```python
from build123d import *

# Parameters (mm, degrees)
BOSS_EXTRUDE1_DEPTH = 6
CUT_EXTRUDE1_DEPTH  = 3.2
SKETCH4_R           = 3
SKETCH4_R_2         = 2
CUT_EXTRUDE2_DEPTH  = 2
SKETCH2_W           = 92.1
SKETCH2_H           = 8
BOSS_EXTRUDE2_DEPTH = 6
FILLET1_R           = 1


with BuildPart() as part:
    # Sketch1 → Boss-Extrude1 (new body)
    with BuildSketch(Plane(origin=(0, 0, 0), x_dir=(1, 0, 0), z_dir=(0, 1, 0))):
        with BuildLine():
            Line((-53.95, 0), (-53.95, 106.281608618))
            ThreePointArc((-53.95, 106.281608618), (-50, 118.95), (-46.05, 106.281608618))
            Line((-46.05, 106.281608618), (-46.05, 0))
            Line((-46.05, 0), (-53.95, 0))
        make_face()
    extrude(amount=BOSS_EXTRUDE1_DEPTH)

    # Sketch3 → Cut-Extrude1 (cut)
    with BuildSketch(Plane.XZ):
        with BuildLine():
            Line((-53.95, -106.281608618), (-53.95, -96.9))
            Line((-53.95, -96.9), (-46.05, -96.9))
            Line((-46.05, -96.9), (-46.05, -106.281608618))
            ThreePointArc((-46.05, -106.281608618), (-50, -118.95), (-53.95, -106.281608618))
        make_face()
    extrude(amount=-CUT_EXTRUDE1_DEPTH, mode=Mode.SUBTRACT)

    # Sketch4 → Cut-Extrude2 (cut)
    with BuildSketch(Plane.XZ.offset(-3.2)):
        with Locations(Location((-50, -112, 0), (0, 0, 270))):
            Circle(SKETCH4_R)
        with Locations(Location((-50, -102, 0), (0, 0, 270))):
            Circle(SKETCH4_R_2)
    extrude(amount=-CUT_EXTRUDE2_DEPTH, mode=Mode.SUBTRACT)


with BuildPart() as body_2:
    # Mirror3: mirrored copy
    add(part.part.mirror(Plane(origin=(0, 0, 0), x_dir=(0, 0, 1), z_dir=(1, 0, 0))))

    # Mirror4 2: body 2 across plane


with BuildPart() as part_1:
    add(part.part)

    # Mirror4: part across plane
    add(part.part.mirror(Plane.XY))



with BuildPart() as body_2_1:
    add(body_2.part)
    add(body_2.part.mirror(Plane.XY))


with BuildPart() as part_2:
    add(part_1.part)

    add(body_2_1.part)  # Boss-Extrude2 merges body 2
    # Sketch2 → Boss-Extrude2 (add)
    with BuildSketch(Plane(origin=(0, 6, 0), x_dir=(1, 0, 0), z_dir=(0, 1, 0))):
        with Locations((0, 54)):
            Rectangle(SKETCH2_W, SKETCH2_H)
        with Locations((0, -54)):
            Rectangle(SKETCH2_W, SKETCH2_H)
    extrude(amount=-BOSS_EXTRUDE2_DEPTH)

    # Fillet1
    fillet1_edges = [part_2.edges().sort_by_distance(p)[0] for p in [
        (-46.05, 0, 0),
        (-46.05, 6, 0),
        (46.05, 3, 50),
        (46.05, 3, 58),
        (-46.05, 3, 58),
        (-46.05, 3, 50),
        (0, 6, 50),
        (0, 6, 58),
        (0, 0, 58),
        (0, 0, 50),
        (-53.95, 0, 0),
        (-53.95, 6, 0),
        (-46.05, 0, 77.45),
        (-46.05, 0, -77.45),
        (-46.05, 6, -82.140804309),
        (-46.05, 3, -50),
        (-46.05, 3, -58),
        (46.05, 3, -58),
        (46.05, 3, -50),
        (0, 6, -50),
        (0, 6, -58),
        (0, 0, -58),
        (0, 0, -50),
        (46.05, 6, -82.140804309),
        (46.05, 6, 82.140804309),
        (53.95, 6, 0),
        (53.95, 0, 0),
        (46.05, 0, 77.45),
        (46.05, 0, -77.45),
        (-46.05, 6, 82.140804309),
        (46.05, 0, 0),
        (46.05, 6, 0),
    ]]
    fillet(fillet1_edges, radius=FILLET1_R)


solid = part_2.part
```
The model under review builds one solid part; all positions refer to its coordinate system, in mm. A direction names the side the tool comes from. Round coordinates to 2 decimals unless told otherwise and drop trailing zeros. Order: outer loops, then holes, each group sorted by start corner. A loop starts at its lowest first (then second) coordinate and runs counter-clockwise, first axis right, second up.
(1) For P1, Ø1, axis at y = 5, z = 6.5, coming from the +X side; P2, Ø2, axis at y = 1, z = 69, coming from the -X side; P3, Ø3, axis at x = 49.5, z = -111.5, coming from the -Y side; P4, Ø8, axis at x = 40.5, z = -85.5, coming from the +Y side, all flat-tipped, find the tip position at first contact; note any pin that passes through.
Working result:
P1: stops at x = 53.95
P2: stops at x = -53.95
P3: stops at y = 5.2
P4: passes through
(2) Tool access review of faces 3 (the face through (-47.3, 0, -13.9)), 4 (the face through (-1, 3, 50)), 5 (the face through (51.774, 4.186, 102.923)), 6 (the face through (-50, 3.2, -108)): name each direction out of +Z, -Z, +X, -X, +Y, -Y from which nothing blocks a thin tool from reaching the whole face with its end or side.
Working result:
face 3: +Z, -Z, +X, -X, -Y
face 4: +Y, -Y
face 5: -Y
face 6: -Z, +X, -X, -Y
(3) Take a section at B-B, the plane x = -33.5. State the section outline as (y, z) points.
Working result:
outline: (0, -57) arc R1 ccw to (1, -58) - (5, -58) arc R1 ccw to (6, -57) - (6, -51) arc R1 ccw to (5, -50) - (1, -50) arc R1 ccw to (0, -51) - close; (0, 51) arc R1 ccw to (1, 50) - (5, 50) arc R1 ccw to (6, 51) - (6, 57) arc R1 ccw to (5, 58) - (1, 58) arc R1 ccw to (0, 57) - close
(4) Take a section at A-A, the plane z = -112. State the section outline as (x, y) points.
Working result:
outline: (-56.95, 3.2) - (-53, 3.2) - (-53, 5.2) - (-47, 5.2) - (-47, 3.2) - (-43.05, 3.2) - (-43.05, 6) - (-56.95, 6) - close; (43.05, 3.2) - (47, 3.2) - (47, 5.2) - (53, 5.2) - (53, 3.2) - (56.95, 3.2) - (56.95, 6) - (43.05, 6) - close
(5) Wall thickness on L1, parallel to X at y = 4.7, z = 102; L2, parallel to Z at x = 50, y = 4.3; L3, parallel to X at y = 4.1, z = 112: over which ranges is each line inside the solid? List them lowest first.
Working result:
L1: x = -53.95 to -52, -48 to -46.05, 46.05 to 48, 52 to 53.95
L2: z = -118.95 to -115, -109 to -104, -100 to 100, 104 to 109, 115 to 118.95
L3: x = -56.95 to -53, -47 to -43.05, 43.05 to 47, 53 to 56.95
(6) Mouldability with a two-part tool opening along Z and no side actions: class faces 1 (the face through (-47.47, 4.19, -113.61)), 2 (the face through (-50, 3.2, 108)) as released by +Z, released by -Z, zero draft, split by the parting line, or undercut.
Working result:
face 1: undercut
face 2: zero draft
